The listing builds one solid part. Answer for the finished solid, in the listing's coordinates (mm). Face numbers are marked on the shaded views. A direction names the side the tool comes from. Give positions to 0.01 mm unless a question says otherwise; leave off trailing zeros. Loops run counter-clockwise (first coordinate to the right, second up) from the corner with the lowest first, then second, coordinate; pieces in that order, holes last. Notation, with made-up numbers: (86.5, 32.25) - (127.5, 32.25) arc R21 cw to (127.5, 46.25) - close; hole circle Ø7 at (34.5, 56). An arc over 180 degrees is marked (long way). Answer as CSV lines item,"result". Start each with the question number.
1) A cutting plane is placed at D-D (z = 25.5). Determine the outline of the cut face in (x, y), and give its area (3 significant figures).
2) A cutting plane is placed at B-B (x = 0). Give the number of separate pieces and of enclosed holes in the cut face, and give its area (3 significant figures).
3) A cutting plane is placed at A-A (z = 19). Determine the outline of the cut face in (x, y).
4) For the marked faces 1, 2 and 3, determine the directions among +Z, -Z, +X, -X, +Y, -Y from which every point of the face is accessible in a straight line to the end or side of a thin tool.
5) Flat-ended cylindrical pins translate along their axes: pin 1 (6 mm diameter, centred on y = -11.68, z = 33.72, fed in from +X); pin 2 (3.5 mm diameter, centred on y = 11.94, z = 6.68, fed in from -X); pin 3 (1 mm diameter, centred on x = 10, z = 17, fed in from +Y); pin 4 (9 mm diameter, centred on y = -11.68, z = 33.72, fed in from -X). Find the tip coordinate at first contact, or state that the pin passes through.
6) For a pull along X with two mould halves and no side action, classify the marked faces 4, 5 and 6 as pulls with the +X half, pulls with the -X half, needs draft (parallel to the pull), parting line crosses it, or undercut.
7) Find the intervals of material crossed by line 1 along Y through (x, z) = (0, 16.5); line 2 along Z through (x, y) = (-14, -6); line 3 along Z through (x, y) = (8, -12), in increasing order.
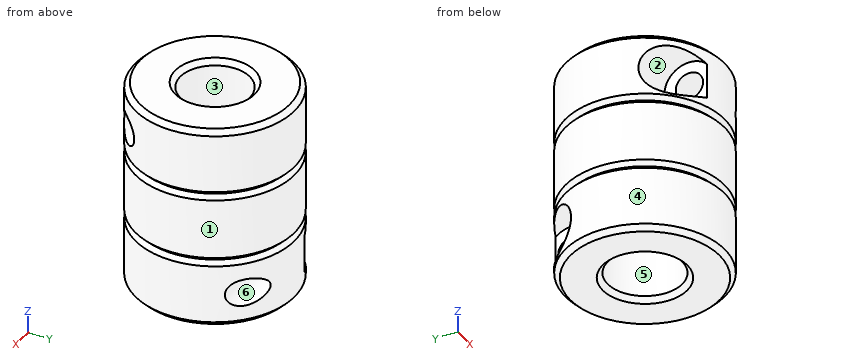
```python
from build123d import *

# Parameters (mm, degrees)
HOLE_WIZARD_M5_1_D           = 5.5
HOLE_WIZARD_M5_1_DEPTH       = 30.416781825
HOLE_WIZARD_M5_1_CBORE_D     = 10
HOLE_WIZARD_M5_1_CBORE_DEPTH = 9.416781825
HOLE_WIZARD_M5_2_D           = 5.5
HOLE_WIZARD_M5_2_DEPTH       = 30.537541482
HOLE_WIZARD_M5_2_CBORE_D     = 10
HOLE_WIZARD_M5_2_CBORE_DEPTH = 9.537541482
HOLE_WIZARD_15_0_15_1_D      = 15
HOLE_WIZARD_15_0_15_1_DEPTH  = 20
HOLE_WIZARD_14_0_14_1_D      = 14
HOLE_WIZARD_14_0_14_1_DEPTH  = 20
CHAMFER_1_SIZE               = 1


with BuildPart() as part:
    # 草图1 → 旋转1 (revolve)
    with BuildSketch(Plane.XZ, mode=Mode.PRIVATE) as revolve_1_sk:
        Polygon((16, 41), (0, 41), (0, 0), (16, 0), (16, 12.716084229), (15.128119248, 13.587964981), (16, 14.459845733), (16, 26.540154267), (15.128119248, 27.412035019), (16, 28.283915771), align=None)
    revolve(revolve_1_sk.sketch.rotate(Axis((0, 0, 41), (0, 0, -1)), 180), axis=Axis((0, 0, 41), (0, 0, -1)))

    # M5 六角头螺栓的柱形沉头孔1
    with Locations(Plane.ZY.offset(14.416781825)):
        with Locations((6.680362699, 11.93948138)):
            CounterBoreHole(HOLE_WIZARD_M5_1_D / 2, HOLE_WIZARD_M5_1_CBORE_D / 2, HOLE_WIZARD_M5_1_CBORE_DEPTH, depth=HOLE_WIZARD_M5_1_DEPTH)

    # M5 六角头螺栓的柱形沉头孔2
    with Locations(Plane.ZY.offset(14.537541482)):
        with Locations((33.720086876, -11.682805373)):
            CounterBoreHole(HOLE_WIZARD_M5_2_D / 2, HOLE_WIZARD_M5_2_CBORE_D / 2, HOLE_WIZARD_M5_2_CBORE_DEPTH, depth=HOLE_WIZARD_M5_2_DEPTH)

    # Ø15.0 (15) 直径孔1
    with Locations(Plane(origin=(0, 0, 0), x_dir=(-1, 0, 0), z_dir=(0, 0, -1))):
        with Locations((0, 0)):
            Hole(HOLE_WIZARD_15_0_15_1_D / 2, depth=HOLE_WIZARD_15_0_15_1_DEPTH)

    # Ø14.0 (14) 直径孔1
    with Locations(Plane.XY.offset(41)):
        with Locations((0, 0)):
            Hole(HOLE_WIZARD_14_0_14_1_D / 2, depth=HOLE_WIZARD_14_0_14_1_DEPTH)

    # 倒角1
    chamfer_1_edges = [part.edges().sort_by_distance(p)[0] for p in [
        (16, 0, 0),
        (16, 0, 41),
        (-7.5, 0, 0),
        (7, 0, 41),
    ]]
    chamfer(chamfer_1_edges, length=CHAMFER_1_SIZE)


solid = part.part
```
Ans:
1,outline,"circle Ø32 at (0, 0); hole circle Ø14 at (0, 0)"
1,area,"650 mm2"
2,separate pieces,"1"
2,enclosed holes,"2"
2,area,"677 mm2"
3,outline,"circle Ø32 at (0, 0); hole circle Ø15 at (0, 0)"
4,face 1,"+Z, -Z"
4,face 2,"-X"
4,face 3,"+Z"
5,pin 1,"x = 13.44"
5,pin 2,"through"
5,pin 3,"y = 12.87"
5,pin 4,"x = -5"
6,face 4,"parting line crosses it"
6,face 5,"undercut"
6,face 6,"needs draft"
7,line 1,"-16 to -7.5, 7.5 to 16"
7,line 2,"0.23 to 13.48, 13.69 to 27.31, 27.52 to 40.77"
7,line 3,"0 to 30.99, 36.45 to 41"
